from build123d import *

# Parameters (mm, degrees)
SKETCH1_R           = 2
BOSS_EXTRUDE1_DEPTH = 1.5


with BuildPart() as part:
    # Sketch1 → Boss-Extrude1 (new body)
    with BuildSketch(Plane.XY):
        with BuildLine():
            Line((12, 8), (12, 1))
            ThreePointArc((12, 1), (11.707106781, 0.292893219), (11, 0))
            Line((11, 0), (1, 0))
            ThreePointArc((1, 0), (0.292893219, 0.292893219), (0, 1))
            Line((0, 1), (0, 94.000005673))
            ThreePointArc((0, 94.000005673), (0.292893219, 94.707112454), (1, 95.000005673))
            Line((1, 95.000005673), (33.760008368, 95.000005673))
            ThreePointArc((33.760008368, 95.000005673), (34.467115149, 94.707112454), (34.760008368, 94.000005673))
            Line((34.760008368, 94.000005673), (34.760008368, 87.000005673))
            ThreePointArc((34.760008368, 87.000005673), (34.467115149, 86.292898892), (33.760008368, 86.000005673))
            Line((33.760008368, 86.000005673), (10, 86.000005673))
            ThreePointArc((10, 86.000005673), (9.292893219, 85.707112454), (9, 85.000005673))
            Line((9, 85.000005673), (9, 10))
            ThreePointArc((9, 10), (9.292893219, 9.292893219), (10, 9))
            Line((10, 9), (11, 9))
            ThreePointArc((11, 9), (11.707106781, 8.707106781), (12, 8))
        make_face()
        with Locations((29.760008368, 90.500005673)):
            Circle(SKETCH1_R, mode=Mode.SUBTRACT)
        with Locations((8, 4.5)):
            Circle(SKETCH1_R, mode=Mode.SUBTRACT)
    extrude(amount=BOSS_EXTRUDE1_DEPTH)


solid = part.part
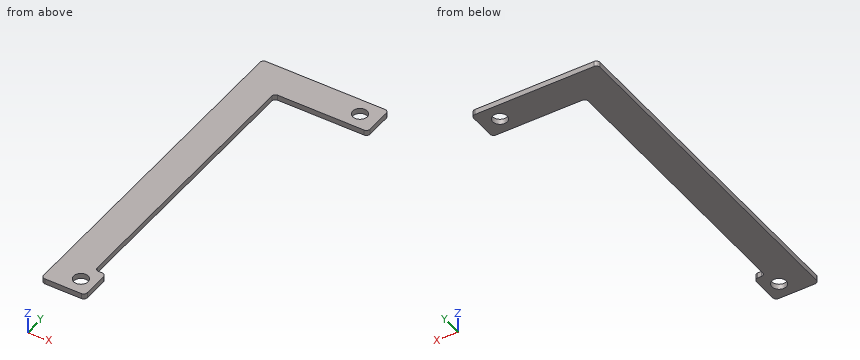
Can you work these out from the model? Positions are in its coordinate system, mm. Round coordinates to 2 decimals unless told otherwise and drop trailing zeros. Write each loop counter-clockwise with the first axis right and the second up, starting at its lowest first coordinate (ties: lowest second). Pieces come first, ordered by that corner, then holes. Notation, with made-up numbers: M 62,-37.5 L 91,-37.5 A27 cw 91,-10.5 Z; hole C 49,15 d5. An arc over 180 degrees is marked long. Use a Markdown table: item, result.
Item 1: For pin 1 Ø12 at (x, y) = (19.5, 71.5) entering from +Z, with a flat end and sliding along its axis, tell me the tip position at first contact or that it passes through.
Found:
| item | result |
|---|---|
| pin 1 | passes through |
Item 2: If I drill on line 1 along Y through (x, z) = (10.5, 0.8); line 2 along Y through (x, z) = (8, 0.6); line 3 along X through (y, z) = (33, 0.5), over which ranges is the centre line in solid material (lowest first)? Write a range as [from, to].
Found:
| item | result |
|---|---|
| line 1 | y = [0, 9], [86, 95] |
| line 2 | y = [0, 2.5], [6.5, 95] |
| line 3 | x = [0, 9] |
Item 3: I want a section at C-C (y = 4.5). List the corners of the cut face in (x, z) for me.
Found:
| item | result |
|---|---|
| outline | M 0,0 L 6,0 L 6,1.5 L 0,1.5 Z; M 10,0 L 12,0 L 12,1.5 L 10,1.5 Z |
Item 4: I want a section at A-A (x = 8). List the corners of the cut face in (y, z) for me, and give its area (4 significant figures).
Found:
| item | result |
|---|---|
| outline | M 0,0 L 2.5,0 L 2.5,1.5 L 0,1.5 Z; M 6.5,0 L 95,0 L 95,1.5 L 6.5,1.5 Z |
| area | 136.5 mm2 |
Item 5: I want a section at D-D (x = 26.5). List the corners of the cut face in (y, z) for me.
Found:
| item | result |
|---|---|
| outline | M 86,0 L 95,0 L 95,1.5 L 86,1.5 Z |
Item 6: I want a section at B-B (z = 0.95). List the corners of the cut face in (x, y) for me, and give its area (3 significant figures).
Found:
| item | result |
|---|---|
| outline | M 0,1 A1 ccw 1,0 L 11,0 A1 ccw 12,1 L 12,8 A1 ccw 11,9 L 10,9 A1 cw 9,10 L 9,85 A1 cw 10,86 L 33.76,86 A1 ccw 34.76,87 L 34.76,94 A1 ccw 33.76,95 L 1,95 A1 ccw 0,94 Z; hole C 8,4.5 d4; hole C 29.76,90.5 d4 |
| area | 1,090 mm2 |
